from build123d import *

# Parameters (mm, degrees)
SKETCH1_W           = 143.51
SKETCH1_H           = 19.05
BOSS_EXTRUDE1_DEPTH = 6.35
SKETCH3_R           = 4.7625
CUT_EXTRUDE1_DEPTH  = 6.35
FILLET5_RADIUS      = 9.525
FILLET5_LENGTH      = 6.35
FILLET6_RADIUS      = 9.525
FILLET6_LENGTH      = 6.35


with BuildPart() as part:
    # Sketch1 → Boss-Extrude1 (new body)
    with BuildSketch(Plane.XY):
        with Locations((9.136619712, 9.525)):
            Rectangle(SKETCH1_W, SKETCH1_H)
    extrude(amount=BOSS_EXTRUDE1_DEPTH)

    # Sketch3 → Cut-Extrude1 (cut)
    with BuildSketch(Plane.XY):
        with Locations((-53.093380288, 9.525)):
            Circle(SKETCH3_R)
        with Locations((71.366619712, 9.525)):
            Circle(SKETCH3_R)
    extrude(amount=CUT_EXTRUDE1_DEPTH, mode=Mode.SUBTRACT)

    # Fillet5: full round fillet: the end face becomes a half cylinder, R = half its width
    fillet5_face = Plane((-62.618380288, 9.525, 3.175), x_dir=(0, 0, -1), z_dir=(-1, 0, 0))  # on the end face: x along it, z out of the body
    fillet5_slab = fillet5_face.offset(-FILLET5_RADIUS / 2) * Box(FILLET5_LENGTH, 2 * FILLET5_RADIUS, FILLET5_RADIUS, mode=Mode.PRIVATE)  # the body's end, R deep
    fillet5_round = Plane((-53.093380288, 9.525, 3.175), x_dir=(-1, 0, 0), z_dir=(0, 0, -1)) * Cylinder(FILLET5_RADIUS, FILLET5_LENGTH, mode=Mode.PRIVATE)  # its axis R under the face
    add(fillet5_slab - fillet5_round, mode=Mode.SUBTRACT)

    # Fillet6: full round fillet: the end face becomes a half cylinder, R = half its width
    fillet6_face = Plane((80.891619712, 9.525, 3.175), x_dir=(0, 0, 1), z_dir=(1, 0, 0))  # on the end face: x along it, z out of the body
    fillet6_slab = fillet6_face.offset(-FILLET6_RADIUS / 2) * Box(FILLET6_LENGTH, 2 * FILLET6_RADIUS, FILLET6_RADIUS, mode=Mode.PRIVATE)  # the body's end, R deep
    fillet6_round = Plane((71.366619712, 9.525, 3.175), x_dir=(1, 0, 0), z_dir=(0, 0, 1)) * Cylinder(FILLET6_RADIUS, FILLET6_LENGTH, mode=Mode.PRIVATE)  # its axis R under the face
    add(fillet6_slab - fillet6_round, mode=Mode.SUBTRACT)


solid = part.part
Read the model definition and answer for the solid it produces. Units are mm, in the model's axes. Give positions to 0.01 mm unless a question says otherwise; leave off trailing zeros. Write each loop counter-clockwise with the first axis right and the second up, starting at its lowest first coordinate (ties: lowest second). Pieces come first, ordered by that corner, then holes. Notation, with made-up numbers: (-36.75, 61.25) - (-17.75, 61.25) arc R11 cw to (-17.75, 71.25) - close; hole circle Ø4 at (42, 9.25). An arc over 180 degrees is marked (long way). Return JSON: item names as keys, results as strings.
Q1. A cutting plane is placed at B-B, the plane y = 8.25. Determine the outline of the cut face in (x, z).
Reply:
{"outline": "(-62.53, 0) - (-57.68, 0) - (-57.68, 6.35) - (-62.53, 6.35) - close; (-48.5, 0) - (66.78, 0) - (66.78, 6.35) - (-48.5, 6.35) - close; (75.96, 0) - (80.81, 0) - (80.81, 6.35) - (75.96, 6.35) - close"}
Q2. Given P1, Ø8.5, axis at x = -53.09, y = 9.52, coming from the -Z side; P2, Ø1.5, axis at y = 14.5, z = 3.5, coming from the +X side; P3, Ø2, axis at y = 8, z = 1, coming from the -X side; P4, Ø2, axis at y = 15.5, z = 2.5, coming from the +X side, each flat-ended and moving along its own axis, determine where each tip first touches the part or whether it passes through.
Reply:
{"P1": "through", "P2": "x = 79.9", "P3": "x = -62.6", "P4": "x = 79.49"}
Q3. Consider line 1 along X through (y, z) = (9.75, 2.5); line 2 along X through (y, z) = (9, 2); line 3 along Y through (x, z) = (72.5, 4). Determine where each line is inside the solid, lowest interval first. Write a range as [from, to].
Reply:
{"line 1": "[-62.62, -57.85], [-48.34, 66.61], [76.12, 80.89]", "line 2": "[-62.6, -57.83], [-48.36, 66.63], [76.1, 80.88]", "line 3": "[0.07, 4.9], [14.15, 18.98]"}
Q4. A cutting plane is placed at D-D, the plane y = 15.5. Determine the outline of the cut face in (x, z), and give its area (3 significant figures).
Reply:
{"outline": "(-60.51, 0) - (78.78, 0) - (78.78, 6.35) - (-60.51, 6.35) - close", "area": "885 mm²"}
Q5. For a pull along X with two mould halves and no side action, classify faces 1 (the face through (-57.85, 9.73, 3.13)), 2 (the face through (8, 10, 6.35)), 3 (the face through (66.61, 9.73, 3.13)), 4 (the face through (-62.616, 9.316, 3.131)) as released by +X, released by -X, zero draft, split by the parting line, or undercut.
Reply:
{"face 1": "undercut", "face 2": "zero draft", "face 3": "undercut", "face 4": "released by -X"}
Q6. A cutting plane is placed at C-C, the plane z = 5. Count the separate pieces of the cut face and the enclosed holes in it, and give its area (3 significant figures).
Reply:
{"separate pieces": "1", "enclosed holes": "2", "area": "2,510 mm²"}
Q7. A cutting plane is placed at A-A, the plane x = -50. Determine the outline of the cut face in (y, z), and give its area (3 significant figures).
Reply:
{"outline": "(0, 0) - (5.9, 0) - (5.9, 6.35) - (0, 6.35) - close; (13.15, 0) - (19.05, 0) - (19.05, 6.35) - (13.15, 6.35) - close", "area": "75.0 mm²"}
